Work out the finished part from the listing and answer in its coordinate system (mm). Face numbers are marked on the shaded views. A direction names the side the tool comes from. Round coordinates to 2 decimals unless told otherwise and drop trailing zeros. Write each loop counter-clockwise with the first axis right and the second up, starting at its lowest first coordinate (ties: lowest second). Pieces come first, ordered by that corner, then holes.
1. A tool of negligible diameter and unlimited length cuts with its end or side. For the marked faces 1 and 2, from which of +Z, -Z, +X, -X, +Y, -Y can it reach the whole face along a straight path? Write none if from no direction.
2. Find section B-B (x = 0). Write down the section's boundary in (y, z).
3. Find section A-A (y = 0). Write down the section's boundary in (x, z).
4. Determine the mould class of the marked faces 3, 4 and 5 for opening direction X: pulls with the +X half, pulls with the -X half, needs draft (parallel to the pull), parting line crosses it, or undercut.
5. Flat-ended cylindrical pins translate along their axes: pin 1 Ø1.5 at (y, z) = (2, -11) entering from +X; pin 2 Ø2 at (y, z) = (7.5, -70.5) entering from +X; pin 3 Ø8 at (x, z) = (5, -24) entering from -Y; pin 4 Ø3 at (x, y) = (-3, -14) entering from +Z. Find the tip coordinate at first contact, or state that the pin passes through.
6. Straight lines are drawn through the part: probe 1 along Z at (x, y) = (0, -1); probe 2 along Z at (x, y) = (-11.5, -3); probe 3 along Z at (x, y) = (3, -6). For each, find the intervals that lie inside material, in ascending order.
7. Find section C-C (z = -51). Write down the section's boundary in (x, y), and give its area (3 significant figures).
8. Find section D-D (z = -75). Write down the section's boundary in (x, y).
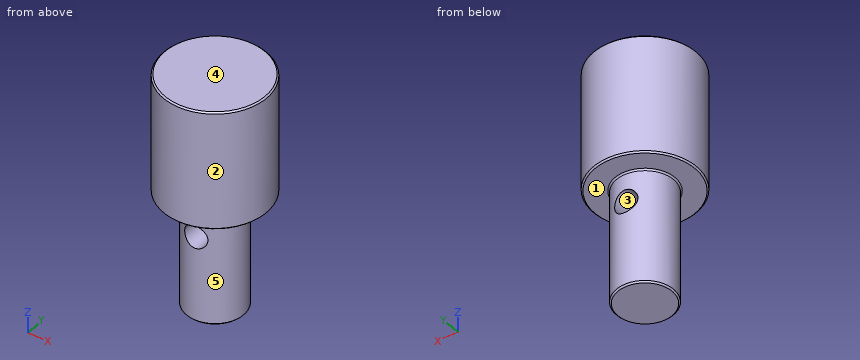
```python
from build123d import *

# Parameters (mm, degrees)
SKETCH_2_R          = 4
CUT_EXTRUDE_1_DEPTH = 89.128088598
FILLET_1_R          = 0.5
CHAMFER_1_SIZE      = 0.5


with BuildPart() as part:
    # Эскиз1 → Повернуть1 (revolve)
    with BuildSketch(Plane(origin=(0, 0, 0), x_dir=(0, 0, -1), z_dir=(1, 0, 0)), mode=Mode.PRIVATE) as revolve_1_sk:
        Polygon((0, 0), (0, 18), (41.6, 18), (41.6, 10), (81.6, 10), (81.6, 0), align=None)
    revolve(revolve_1_sk.sketch.rotate(Axis((0, 0, 0), (0, 0, -1)), 180), axis=Axis((0, 0, 0), (0, 0, -1)))

    # Эскиз2 → Вырез-Вытянуть1 (cut, through all)
    with BuildSketch(Plane(origin=(0, 10, 0), x_dir=(1, 0, 0), z_dir=(0, 1, 0))):
        with Locations(Location((0, 51.6, 0), (0, 0, 269.999999991))):
            Circle(SKETCH_2_R)
    extrude(amount=-CUT_EXTRUDE_1_DEPTH, mode=Mode.SUBTRACT)

    # Скругление1
    fillet_1_edges = [part.edges().sort_by_distance(p)[0] for p in [
        (0, 10, -41.6),
    ]]
    fillet(fillet_1_edges, radius=FILLET_1_R)

    # Фаска1
    chamfer_1_edges = [part.edges().sort_by_distance(p)[0] for p in [
        (0, 10, -81.6),
        (0, 18, -41.6),
        (0, 18, 0),
    ]]
    chamfer(chamfer_1_edges, length=CHAMFER_1_SIZE)


solid = part.part
```
Worked answers:
1. face 1: -Z
1. face 2: +Z, -Z
2. outline: (-18, -41.1) - (-17.5, -41.6) - (-10.5, -41.6) arc R0.5 cw to (-10, -42.1) - (-10, -47.6) - (10, -47.6) - (10, -42.1) arc R0.5 cw to (10.5, -41.6) - (17.5, -41.6) - (18, -41.1) - (18, -0.5) - (17.5, 0) - (-17.5, 0) - (-18, -0.5) - close; (-10, -81.1) - (-9.5, -81.6) - (9.5, -81.6) - (10, -81.1) - (10, -55.6) - (-10, -55.6) - close
3. outline: (-18, -41.1) - (-17.5, -41.6) - (-10.5, -41.6) arc R0.5 cw to (-10, -42.1) - (-10, -81.1) - (-9.5, -81.6) - (9.5, -81.6) - (10, -81.1) - (10, -42.1) arc R0.5 cw to (10.5, -41.6) - (17.5, -41.6) - (18, -41.1) - (18, -0.5) - (17.5, 0) - (-17.5, 0) - (-18, -0.5) - close; hole circle Ø8 at (0, -51.6)
4. face 3: undercut
4. face 4: needs draft
4. face 5: parting line crosses it
5. pin 1: stops at x = 17.96
5. pin 2: stops at x = 7.6
5. pin 3: stops at y = -17.97
5. pin 4: stops at z = 0
6. probe 1: z = -81.6 to -55.6, -47.6 to 0
6. probe 2: z = -41.6 to 0
6. probe 3: z = -81.6 to -54.25, -48.95 to 0
7. outline: (-3.95, -9.18) - (-3.95, 9.18) arc R10 ccw to start; (3.95, -9.18) arc R10 ccw to (3.95, 9.18) - close
7. area: 160 mm2
8. outline: circle Ø20 at (0, 0)
